For this review, use the dimensioned drawing (mm, ordinates from the lowest corner) and the shaded views. A direction names the side the tool comes from. Coordinates: 2 decimals unless noted, no trailing zeros. Loops run counter-clockwise (first coordinate to the right, second up) from the corner with the lowest first, then second, coordinate; pieces in that order, holes last.
1. Take a section at A-A, the plane z = 3.2. State the section outline as (x, y) points, then the cut area to 3 significant figures.
2. Take a section at C-C, the plane z = 1.7. State the section outline as (x, y) points.
3. Mouldability with a two-part tool opening along Y and no side actions: class the marked faces 1, 2, 3 and 4 as pulls with the +Y half, pulls with the -Y half, needs draft (parallel to the pull), parting line crosses it, or undercut.
4. Take a section at D-D, the plane x = 4.75. State the section outline as (y, z) points.
5. Clearance check with flat-ended pins moving along their axes: P1, Ø1, axis at y = 10.5, z = 3, coming from the +X side; P2, Ø1, axis at x = 4, z = 3.5, coming from the -Y side; P3, Ø1, axis at x = 8.5, z = 3.5, coming from the +Y side; P4, Ø1.6, axis at x = 6, z = 2.5, coming from the +Y side. State where each tip first meets the part, or that it passes through.
6. Machinability: for the marked faces 5, 6, 7, 8 and 9, which of the approach directions +Z, -Z, +X, -X, +Y, -Y give a long, thin tool a straight path to every point of the face, cutting with its end or side? Answer none if there is none.
7. Take a section at B-B, the plane x = 9.75. State the section outline as (y, z) points.
8. To check wall thickness, follow probe 1 along Y at (x, z) = (8.5, 2.3); probe 2 along X at (y, z) = (10.5, 3.6); probe 3 along X at (y, z) = (2, 3.65). State the ranges of each line that lie inside material, in increasing order.
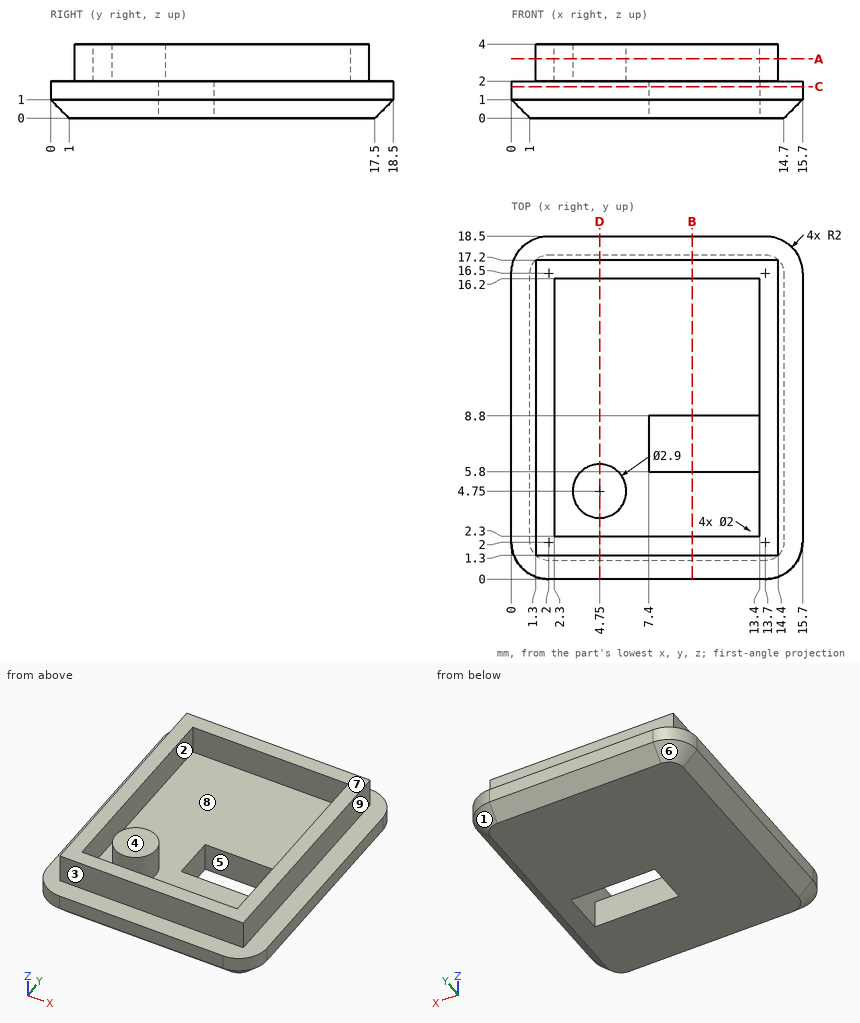
Results list:
1. outline: (1.3, 1.3) - (14.4, 1.3) - (14.4, 17.2) - (1.3, 17.2) - close; circle Ø2.9 at (4.75, 4.75); hole (2.3, 2.3) - (13.4, 2.3) - (13.4, 16.2) - (2.3, 16.2) - close
1. area: 60.6 mm2
2. outline: (0, 2) arc R2 ccw to (2, 0) - (13.7, 0) arc R2 ccw to (15.7, 2) - (15.7, 16.5) arc R2 ccw to (13.7, 18.5) - (2, 18.5) arc R2 ccw to (0, 16.5) - close; hole (7.4, 5.8) - (13.4, 5.8) - (13.4, 8.8) - (7.4, 8.8) - close
3. face 1: pulls with the +Y half
3. face 2: undercut
3. face 3: pulls with the -Y half
3. face 4: needs draft
4. outline: (0, 1) - (1, 0) - (17.5, 0) - (18.5, 1) - (18.5, 2) - (17.2, 2) - (17.2, 4) - (16.2, 4) - (16.2, 2) - (6.2, 2) - (6.2, 4) - (3.3, 4) - (3.3, 2) - (2.3, 2) - (2.3, 4) - (1.3, 4) - (1.3, 2) - (0, 2) - close
5. P1: stops at x = 14.4
5. P2: stops at y = 1.3
5. P3: stops at y = 17.2
5. P4: stops at y = 18.5
6. face 5: +Z, -Z
6. face 6: -Z, -X, +Y
6. face 7: +Z, +X, -X, +Y, -Y
6. face 8: +Z
6. face 9: +Z, +X, +Y, -Y
7. outline: (0, 1) - (1, 0) - (5.8, 0) - (5.8, 2) - (2.3, 2) - (2.3, 4) - (1.3, 4) - (1.3, 2) - (0, 2) - close; (8.8, 0) - (17.5, 0) - (18.5, 1) - (18.5, 2) - (17.2, 2) - (17.2, 4) - (16.2, 4) - (16.2, 2) - (8.8, 2) - close
8. probe 1: y = 1.3 to 2.3, 16.2 to 17.2
8. probe 2: x = 1.3 to 2.3, 13.4 to 14.4
8. probe 3: x = 1.3 to 14.4
